```python
from build123d import *

# Parameters (mm, degrees)
F1_DEPTH  = 12
F2_R      = 11.1
F3_DEPTH  = 12.001
F5_R      = 2.1
F6_DEPTH  = 12.001
F7_R      = 4
F8_DEPTH  = 3
F9_R      = 4
F10_DEPTH = 3
F11_R     = 7.5
F12_DEPTH = 12.001


with BuildPart() as f1:
    # F0 (on Top) → F1 (new body)
    with BuildSketch(Plane.XY):
        Polygon((60.5, -30), (72.5, -30), (72.5, 30), (60.5, 30), (60.5, 16), (60.5, -16), align=None)
        Polygon((-72.5, -11), (60.5, -16), (60.5, 16), (-72.5, 11), align=None)
    extrude(amount=F1_DEPTH)

    # F2 (on face) → F3 (cut, through all)
    with BuildSketch(Plane.XY.offset(12)):
        with Locations((-51.4, 11.793233)):
            Circle(F2_R)
    extrude(amount=-F3_DEPTH, mode=Mode.SUBTRACT)

    # F5 (on offset) → F6 (cut, through all)
    with BuildSketch(Plane.YZ.offset(60.5)):
        with Locations((24, 6)):
            Circle(F5_R)
        with Locations((-24, 6)):
            Circle(F5_R)
    extrude(amount=F6_DEPTH, mode=Mode.SUBTRACT)

    # F7 (on face) → F8 (cut)
    with BuildSketch(Plane(origin=(60.5, 0, 0), x_dir=(0, -1, 0), z_dir=(-1, 0, 0))):
        with Locations((-24, 6)):
            Circle(F7_R)
    extrude(amount=-F8_DEPTH, mode=Mode.SUBTRACT)

    # F9 (on face) → F10 (cut)
    with BuildSketch(Plane(origin=(60.5, 0, 0), x_dir=(0, -1, 0), z_dir=(-1, 0, 0))):
        with Locations((24, 6)):
            Circle(F9_R)
    extrude(amount=-F10_DEPTH, mode=Mode.SUBTRACT)

    # F11 (on face) → F12 (cut, through all)
    with BuildSketch(Plane.XY.offset(12)):
        with Locations((-30, 0)):
            Circle(F11_R)
        with Locations((-10, 0)):
            Circle(F11_R)
        with Locations((10, 0)):
            Circle(F11_R)
        with Locations((30, 0)):
            Circle(F11_R)
        with Locations((50, 0)):
            Circle(F11_R)
    extrude(amount=-F12_DEPTH, mode=Mode.SUBTRACT)


solid = f1.part
```
Check sheet for the modelled part. Datum: model origin and axes. Units: mm. A direction names the side the tool comes from. Round coordinates to 2 decimals unless told otherwise and drop trailing zeros. Write each loop counter-clockwise with the first axis right and the second up, starting at its lowest first coordinate (ties: lowest second). Pieces come first, ordered by that corner, then holes. Notation, with made-up numbers: M 40,22.5 L 94,22.5 A16 ccw 94,49.5 Z; hole C 69,-4 d6. An arc over 180 degrees is marked long. Write item = value, one per line. Start each with the question number.
1. Gauge pin test, flat ends, axial feed: pin 1 (1.5 mm diameter, centred on x = 57.5, z = 1, fed in from -Y); pin 2 (1 mm diameter, centred on x = -52, z = 3.5, fed in from +Y); pin 3 (2.5 mm diameter, centred on y = -24.5, z = 4, fed in from -X); pin 4 (19.5 mm diameter, centred on x = 10, y = 0, fed in from -Z). Record the tip position at first contact, or that the pin passes through.
2. Section check B-B, the plane y = -24. Record the cut outline in (x, z), then the cut area to 3 significant figures.
3. Section check A-A, the plane z = 6. State how many separate pieces and enclosed holes the cut face has, then the cut area to 3 significant figures.
4. Tool access check on faces 4 (the flat face through (63.5, -26, 4)), 5 (the cylindrical face through (57.154, 2.253, 6.084)), 6 (the flat face through (60.5, 20, 4.6)). Record the directions out of +Z, -Z, +X, -X, +Y, -Y that give a thin tool (end or side, any length) a straight path to the whole face; none if there is none.
5. Section check D-D, the plane y = 4.5. Record the cut outline in (x, z).
6. Scan lines: line 1 (X direction, y = 0.5, z = 8.5); line 2 (Z direction, x = 61, y = 24); line 3 (Y direction, x = 30, z = 1.5). Record each from-to range of solid material in increasing order. Write a range as [from, to].
7. Section check C-C, the plane x = 46. Record the cut outline in (y, z), then the cut area to 3 significant figures.
8. Release check for a two-part mould opening along X. For faces 1 (the cylindrical face through (-37.493, 0.33, 6.084)), 2 (the flat face through (60.5, -19.8, 5.9)), 3 (the flat face through (66, -30, 6)) record: pulls with the +X half, pulls with the -X half, needs draft (parallel to the pull), parting line crosses it, or undercut.
Results found:
q1.pin_1 = -15.92
q1.pin_2 = 0.75
q1.pin_3 = 63.5
q1.pin_4 = 0
q2.outline = M 60.5,0 L 72.5,0 L 72.5,3.9 L 63.5,3.9 L 63.5,2 L 60.5,2 Z; M 60.5,10 L 63.5,10 L 63.5,8.1 L 72.5,8.1 L 72.5,12 L 60.5,12 Z
q2.area = 82.2 mm^2
q3.separate_pieces = 3
q3.enclosed_holes = 5
q3.area = 3,110 mm^2
q4.face_4 = -X
q4.face_5 = +Z, -Z
q4.face_6 = +Z, -Z, -X, +Y
q5.outline = M -72.5,0 L -59.77,0 L -59.77,12 L -72.5,12 Z; M -43.03,0 L -36,0 L -36,12 L -43.03,12 Z; M -24,0 L -16,0 L -16,12 L -24,12 Z; M -4,0 L 4,0 L 4,12 L -4,12 Z; M 16,0 L 24,0 L 24,12 L 16,12 Z; M 36,0 L 44,0 L 44,12 L 36,12 Z; M 56,0 L 72.5,0 L 72.5,12 L 56,12 Z
q6.line_1 = [-72.5, -37.48], [-22.52, -17.48], [-2.52, 2.52], [17.48, 22.52], [37.48, 42.52], [57.48, 72.5]
q6.line_2 = [0, 2], [10, 12]
q6.line_3 = [-14.85, -7.5], [7.5, 14.85]
q7.outline = M -15.45,0 L -6.34,0 L -6.34,12 L -15.45,12 Z; M 6.34,0 L 15.45,0 L 15.45,12 L 6.34,12 Z
q7.area = 219 mm^2
q8.face_1 = undercut
q8.face_2 = pulls with the -X half
q8.face_3 = needs draft
